```python
from build123d import *

# Parameters (mm, degrees)
BOSS_EXTRUDE1_DEPTH = 57.5
SKETCH2_R           = 7.5
CUT_EXTRUDE1_DEPTH  = 51
SKETCH3_R           = 5
BOSS_EXTRUDE2_DEPTH = 25


with BuildPart() as part:
    # Sketch1 → Boss-Extrude1 (new body, symmetric)
    with BuildSketch(Plane.XY):
        Polygon((0, 150), (0, 0), (50, 0), (50, 10), (10, 10), (10, 150), align=None)
    extrude(amount=BOSS_EXTRUDE1_DEPTH, both=True)

    # Sketch2 → Cut-Extrude1 (cut, through all)
    with BuildSketch(Plane.ZY):
        with Locations((0, 60)):
            Circle(SKETCH2_R)
    extrude(amount=-CUT_EXTRUDE1_DEPTH, mode=Mode.SUBTRACT)

    # Sketch3 → Boss-Extrude2 (add)
    with BuildSketch(Plane(origin=(10, 0, 0), x_dir=(0, 0, -1), z_dir=(1, 0, 0))):
        with Locations((0, 130)):
            Circle(SKETCH3_R)
    extrude(amount=BOSS_EXTRUDE2_DEPTH)


solid = part.part
```
Check sheet for the modelled part. Datum: model origin and axes. Units: mm. A direction names the side the tool comes from. Coordinates: 2 decimals unless noted, no trailing zeros. Loops run counter-clockwise (first coordinate to the right, second up) from the corner with the lowest first, then second, coordinate; pieces in that order, holes last.
1) Access from +Z, -Z, +X, -X, +Y, -Y to the whole of each face (thin tool, end or side, straight path). Record for faces 1 (the face through (8, 59, 57.5)), 2 (the face through (22.325, 134.957, 0.651)), 3 (the face through (35, 130, 0)).
2) Release check for a two-part mould opening along Y. For faces 4 (the face through (4.93, 67.436, -0.976)), 5 (the face through (25, 0, 1)), 6 (the face through (0, 76, 1)) record: released by +Y, released by -Y, zero draft, split by the parting line, or undercut.
3) Sectioned sample at A-A (x = 12). Record the boundary of the cut face in (y, z).
4) Material ranges on probe 1 along Y at (x, z) = (6, 0); probe 2 along X at (y, z) = (106.5, 16.5), recorded low to high.
5) Sectioned sample at C-C (y = 60). Record the boundary of the cut face in (x, z), and give its area (3 significant figures).
6) Sectioned sample at B-B (z = 0). Record the boundary of the cut face in (x, y), and give its area (3 significant figures).
7) Sectioned sample at D-D (y = 130). Record the boundary of the cut face in (x, z), and give its area (3 significant figures).
8) Gauge pin test, flat ends, axial feed: pin 1 (11 mm diameter, centred on y = 129.5, z = 1, fed in from +X); pin 2 (12 mm diameter, centred on x = 30.5, z = 2, fed in from +Y); pin 3 (1 mm diameter, centred on y = 16, z = 37, fed in from +X). Record the tip position at first contact, or that the pin passes through.
Check sheet entries:
1. face 1: +Z, +X, -X, +Y, -Y
1. face 2: +X
1. face 3: +Z, -Z, +X, +Y
2. face 4: undercut
2. face 5: released by -Y
2. face 6: zero draft
3. outline: (0, -57.5) - (10, -57.5) - (10, 57.5) - (0, 57.5) - close; circle Ø10 at (130, 0)
4. probe 1: y = 0 to 52.5, 67.5 to 150
4. probe 2: x = 0 to 10
5. outline: (0, -57.5) - (10, -57.5) - (10, -7.5) - (0, -7.5) - close; (0, 7.5) - (10, 7.5) - (10, 57.5) - (0, 57.5) - close
5. area: 1,000 mm2
6. outline: (0, 0) - (50, 0) - (50, 10) - (10, 10) - (10, 52.5) - (0, 52.5) - close; (0, 67.5) - (10, 67.5) - (10, 125) - (35, 125) - (35, 135) - (10, 135) - (10, 150) - (0, 150) - close
6. area: 2,000 mm2
7. outline: (0, -57.5) - (10, -57.5) - (10, -5) - (35, -5) - (35, 5) - (10, 5) - (10, 57.5) - (0, 57.5) - close
7. area: 1,400 mm2
8. pin 1: stops at x = 35
8. pin 2: stops at y = 135
8. pin 3: stops at x = 10
